from build123d import *

# Parameters (mm, degrees)
SKETCH1_R           = 2.000000064
BOSS_EXTRUDE1_DEPTH = 71.4121
SKETCH4_R           = 6.35
SKETCH4_R_2         = 2.000000064
BOSS_EXTRUDE2_DEPTH = 7.9375


with BuildPart() as part:
    # Sketch1 → Boss-Extrude1 (new, symmetric)
    with BuildSketch(Plane.XY):
        with BuildLine():
            ThreePointArc((4.181770846, 5.456960429), (3.437499983, 5.953924622), (2.634980936, 6.35))
            Line((2.634980936, 6.35), (-2.634980936, 6.35))
            ThreePointArc((-2.634980936, 6.35), (-3.437499983, 5.953924622), (-4.181770846, 5.456960429))
            Line((-4.181770846, 5.456960429), (-6.816751782, 0.893039571))
            ThreePointArc((-6.816751782, 0.893039571), (-6.874999966, 0), (-6.816751782, -0.893039571))
            Line((-6.816751782, -0.893039571), (-4.181770846, -5.456960429))
            ThreePointArc((-4.181770846, -5.456960429), (-3.437499983, -5.953924622), (-2.634980936, -6.35))
            Line((-2.634980936, -6.35), (2.634980936, -6.35))
            ThreePointArc((2.634980936, -6.35), (3.437499983, -5.953924622), (4.181770846, -5.456960429))
            Line((4.181770846, -5.456960429), (6.816751782, -0.893039571))
            ThreePointArc((6.816751782, -0.893039571), (6.860422465, -0.447468582), (6.874999966, 0))
            ThreePointArc((6.874999966, 0), (6.860422465, 0.447468582), (6.816751782, 0.893039571))
            Line((6.816751782, 0.893039571), (4.181770846, 5.456960429))
        make_face()
        Circle(SKETCH1_R, mode=Mode.SUBTRACT)
    extrude(amount=BOSS_EXTRUDE1_DEPTH, both=True)

    # Sketch4 → Boss-Extrude2 (add)
    with BuildSketch(Plane.XY.offset(71.4121)):
        with Locations(Location((0, 0, 0), (0, 0, 150))):
            Circle(SKETCH4_R)
        Circle(SKETCH4_R_2, mode=Mode.SUBTRACT)
    boss_extrude2 = extrude(amount=BOSS_EXTRUDE2_DEPTH)

    # Mirror1: Boss-Extrude2 across plane
    add(boss_extrude2.mirror(Plane.XY))


solid = part.part
The model under review builds one solid part; all positions refer to its coordinate system, in mm. A direction names the side the tool comes from. Coordinates: 2 decimals unless noted, no trailing zeros. Loops run counter-clockwise (first coordinate to the right, second up) from the corner with the lowest first, then second, coordinate; pieces in that order, holes last. Notation, with made-up numbers: (-4, -3.75) -> (54, -3.75) arc R31 ccw to (54, 28.25) -> close; hole circle Ø7 at (8, 80.5). An arc over 180 degrees is marked (long way). Use a Markdown table: item, result. Add a question column.
1. To check wall thickness, follow line 1 (X direction, y = 3.25, z = 39); line 2 (X direction, y = -1.75, z = 40.5); line 3 (X direction, y = 5.5, z = 65.5) (3 decimals). State the ranges of each line that lie inside material, in increasing order.
2. Machinability: for faces 4 (the face through (-3, 6, -71.412)), 5 (the face through (3, 6, -71.412)), 6 (the face through (-3, 6, 71.412)), 7 (the face through (4.29, 4.68, 75.33)), 8 (the face through (-3, -6, 71.412)), which of the approach directions +Z, -Z, +X, -X, +Y, -Y give a long, thin tool a straight path to every point of the face, cutting with its end or side? Answer none if there is none.
3. Add section A-A on z = 50. Write out the cut boundary in (x, y) (3 decimals).
4. Draft analysis for pull direction X (two halves, no side actions). For faces 1 (the face through (-5.52, -3.14, 1)), 2 (the face through (1.908, 0.601, 1.111)), 3 (the face through (3, -6, -71.412)), state which applies: pulls with the +X half, pulls with the -X half, needs draft (parallel to the pull), parting line crosses it, or undercut.
5. Clearance check with flat-ended pins moving along their axes: pin 1 Ø6 at (y, z) = (4.5, 13) entering from +X; pin 2 Ø3.5 at (x, y) = (0, 0) entering from +Z. State where each tip first meets the part, or that it passes through.
Returned:
| question | item | result |
|---|---|---|
| 1 | line 1 | x = -5.46 to 5.46 |
| 1 | line 2 | x = -6.32 to -0.97, 0.97 to 6.32 |
| 1 | line 3 | x = -4.125 to 4.125 |
| 2 | face 4 | -Z, -X, +Y |
| 2 | face 5 | -Z, +X, +Y |
| 2 | face 6 | +Z, -X, +Y |
| 2 | face 7 | +Z |
| 2 | face 8 | +Z, -X, -Y |
| 3 | outline | (-6.817, -0.893) -> (-4.182, -5.457) arc R6.875 ccw to (-2.635, -6.35) -> (2.635, -6.35) arc R6.875 ccw to (4.182, -5.457) -> (6.817, -0.893) arc R6.875 ccw to (6.817, 0.893) -> (4.182, 5.457) arc R6.875 ccw to (2.635, 6.35) -> (-2.635, 6.35) arc R6.875 ccw to (-4.182, 5.457) -> (-6.817, 0.893) arc R6.875 ccw to start; hole circle Ø4 at (0, 0) |
| 4 | face 1 | pulls with the -X half |
| 4 | face 2 | undercut |
| 4 | face 3 | needs draft |
| 5 | pin 1 | stops at x = 6.47 |
| 5 | pin 2 | passes through |
